```python
from build123d import *
from build123d.topology import SkipClean

# Parameters (mm, degrees)
SKETCH_1_W          = 100
SKETCH_1_H          = 18
SKETCH_1_R          = 2.6
SKETCH_1_R_2        = 2
SKETCH_1_R_3        = 1.5
EXTRUDE_1_DEPTH     = 10
SKETCH_2_W          = 70
SKETCH_2_H          = 18
CUT_EXTRUDE_1_DEPTH = 2
FILLET_1_R          = 1.5
EXTRUDE_3_DEPTH     = 2
SKETCH_4_R          = 4
EXTRUDE_4_DEPTH     = 1
SKETCH_5_R          = 3.38932831
EXTRUDE_5_DEPTH     = 3.2
SKETCH_6_R          = 3.75
EXTRUDE_6_DEPTH     = 3.2
SKETCH_7_R          = 3.75
EXTRUDE_7_DEPTH     = 3.2
SKETCH_8_R          = 3.75
EXTRUDE_8_DEPTH     = 3.2
CUT_EXTRUDE_2_DEPTH = 1
CUT_EXTRUDE_3_DEPTH = 1
CUT_EXTRUDE_4_DEPTH = 1


with BuildPart() as part:
    # Эскиз1 → Вытянуть1 (new body)
    with BuildSketch(Plane.XY):
        with Locations((50, 9)):
            Rectangle(SKETCH_1_W, SKETCH_1_H)
        with Locations((7.5, 9)):
            Circle(SKETCH_1_R, mode=Mode.SUBTRACT)
        with Locations((92.5, 9)):
            Circle(SKETCH_1_R, mode=Mode.SUBTRACT)
        with Locations((20, 4)):
            Circle(SKETCH_1_R_2, mode=Mode.SUBTRACT)
        with Locations((80, 4)):
            Circle(SKETCH_1_R_2, mode=Mode.SUBTRACT)
        with Locations((30, 14)):
            Circle(SKETCH_1_R_3, mode=Mode.SUBTRACT)
        with Locations((70, 14)):
            Circle(SKETCH_1_R_3, mode=Mode.SUBTRACT)
    extrude(amount=EXTRUDE_1_DEPTH)

    # Эскиз2 → Вырез-Вытянуть1 (cut)
    with BuildSketch(Plane(origin=(0, 0, 0), x_dir=(-1, 0, 0), z_dir=(0, 0, -1))):
        with Locations((-50, 9)):
            Rectangle(SKETCH_2_W, SKETCH_2_H)
    extrude(amount=-CUT_EXTRUDE_1_DEPTH, mode=Mode.SUBTRACT)

    # Скругление1
    fillet_1_edges = [part.edges().sort_by_distance(p)[0] for p in [
        (100, 0, 5),
        (0, 0, 5),
        (100, 18, 5),
        (0, 18, 5),
    ]]
    fillet(fillet_1_edges, radius=FILLET_1_R)

    # Эскиз3 → Вытянуть3 (add)
    with BuildSketch(Plane.XY.offset(10)):
        with BuildLine():
            Line((72.692526424, 16.844371856), (82.811526632, 6.845227231))
            ThreePointArc((82.811526632, 6.845227231), (82.845227231, 1.188473368), (77.188473368, 1.154772769))
            Line((77.188473368, 1.154772769), (77.139063674, 1.203597224))
            Line((77.139063674, 1.203597224), (22.860092921, 1.203597224))
            ThreePointArc((22.860092921, 1.203597224), (17.203597224, 1.139907079), (17.139907079, 6.796402776))
            Line((17.139907079, 6.796402776), (26.916385172, 16.795547401))
            ThreePointArc((26.916385172, 16.795547401), (32.572880868, 16.859237546), (32.636571013, 11.20274185))
            Line((32.636571013, 11.20274185), (29.016893244, 7.500623237))
            Line((29.016893244, 7.500623237), (70.766557833, 7.500623237))
            Line((70.766557833, 7.500623237), (67.06947316, 11.153917394))
            ThreePointArc((67.06947316, 11.153917394), (67.035772561, 16.810671257), (72.692526424, 16.844371856))
        make_face()
    extrude(amount=EXTRUDE_3_DEPTH)

    # Эскиз4 → Вытянуть4 (add)
    with SkipClean():  # the faces are left unmerged after this step: merging them gives an invalid solid
        with BuildSketch(Plane.XY.offset(12)):
            with Locations(Location((20, 4, 0), (0, 0, 135.645102996))):
                Circle(SKETCH_4_R)
            with Locations(Location((29.776478092, 13.999144625, 0), (0, 0, 135.645102996))):
                Circle(SKETCH_4_R)
            with Locations(Location((69.880999792, 13.999144625, 0), (0, 0, 225.341340509))):
                Circle(SKETCH_4_R)
            with Locations(Location((80, 4, 0), (0, 0, 225.341340509))):
                Circle(SKETCH_4_R)
        extrude(amount=EXTRUDE_4_DEPTH)
    add(part.part.scale(1), mode=Mode.REPLACE)  # the faces are merged on a copy

    # Эскиз5 → Вытянуть5 (add)
    with BuildSketch(Plane.XY.offset(13)):
        with Locations(Location((80, 4, 0), (0, 0, 143.222791585))):
            Circle(SKETCH_5_R)
    extrude(amount=EXTRUDE_5_DEPTH)

    # Эскиз6 → Вытянуть6 (add)
    with BuildSketch(Plane.XY.offset(13)):
        with Locations(Location((69.880999792, 13.999144625, 0), (0, 0, 141.123198866))):
            Circle(SKETCH_6_R)
    extrude(amount=EXTRUDE_6_DEPTH)

    # Эскиз7 → Вытянуть7 (add)
    with BuildSketch(Plane.XY.offset(13)):
        with Locations(Location((29.776478092, 13.999144625, 0), (0, 0, 141.123198866))):
            Circle(SKETCH_7_R)
    extrude(amount=EXTRUDE_7_DEPTH)

    # Эскиз8 → Вытянуть8 (add)
    with BuildSketch(Plane.XY.offset(13)):
        with Locations(Location((20, 4, 0), (0, 0, 141.123198866))):
            Circle(SKETCH_8_R)
    extrude(amount=EXTRUDE_8_DEPTH)

    # Эскиз9 → Вырез-Вытянуть2 (cut)
    with BuildSketch(Plane.XY.offset(16.2)):
        Polygon((16.157845588, 7.276468987), (24.091280084, -0.656965509), (24.596689062, -0.031003637), (16.723531013, 7.842154412), align=None)
    extrude(amount=-CUT_EXTRUDE_2_DEPTH, mode=Mode.SUBTRACT)

    # Эскиз10 → Вырез-Вытянуть3 (cut)
    with BuildSketch(Plane.XY.offset(16.2)):
        Polygon((23.332366462, 19.877570831), (34.653872269, 8.556065024), (35.333565103, 9.007743039), (23.898051887, 20.443256256), align=None)
    extrude(amount=-CUT_EXTRUDE_3_DEPTH, mode=Mode.SUBTRACT)

    # Эскиз11 → Вырез-Вытянуть4 (cut)
    with BuildSketch(Plane.XY.offset(16.2)):
        Polygon((62.841835451, 20.472623541), (84.739405762, -1.42494677), (85.695784292, -1.249954449), (63.522860335, 20.922969507), align=None)
    extrude(amount=-CUT_EXTRUDE_4_DEPTH, mode=Mode.SUBTRACT)


solid = part.part
```
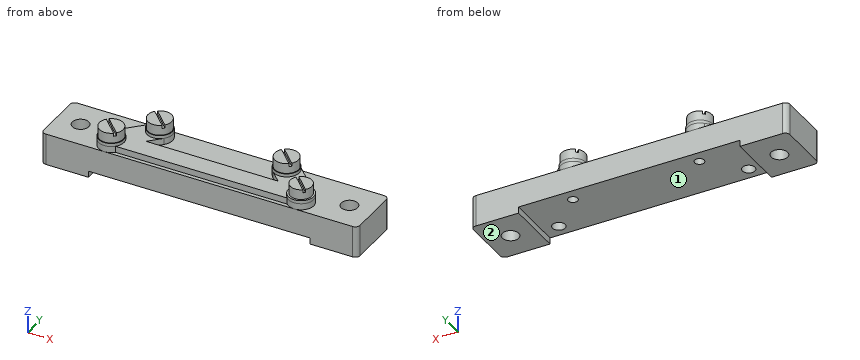
Work out the finished part from the listing and answer in its coordinate system (mm). Face numbers are marked on the shaded views. A direction names the side the tool comes from. Give positions to 0.01 mm unless a question says otherwise; leave off trailing zeros. Write each loop counter-clockwise with the first axis right and the second up, starting at its lowest first coordinate (ties: lowest second). Pieces come first, ordered by that corner, then holes.
(1) Straight lines are drawn through the part: line 1 (X direction, y = 4, z = 8.75); line 2 (X direction, y = 14.25, z = 7.75); line 3 (Y direction, x = 30, z = 6.5). For each, find the intervals that lie inside material, in ascending order.
Final values:
line 1: x = 0 to 18, 22 to 78, 82 to 100
line 2: x = 0 to 28.52, 31.48 to 68.52, 71.48 to 100
line 3: y = 0 to 12.5, 15.5 to 18
(2) Flat-ended cylindrical pins translate along their axes: pin 1 Ø0.9 at (x, y) = (70, 14.5) entering from -Z; pin 2 Ø4.5 at (x, y) = (51.5, 7.5) entering from +Z; pin 3 Ø4.5 at (x, y) = (20.5, 5) entering from -Z. Find the tip coordinate at first contact, or state that the pin passes through.
Final values:
pin 1: stops at z = 10
pin 2: stops at z = 12
pin 3: stops at z = 2
(3) The part is cut by section B-B on z = 8.5. Write down the section's boundary in (x, y), plus the area to 3 significant figures.
Final values:
outline: (0, 1.5) arc R1.5 ccw to (1.5, 0) - (98.5, 0) arc R1.5 ccw to (100, 1.5) - (100, 16.5) arc R1.5 ccw to (98.5, 18) - (1.5, 18) arc R1.5 ccw to (0, 16.5) - close; hole circle Ø5.2 at (7.5, 9); hole circle Ø4 at (20, 4); hole circle Ø3 at (30, 14); hole circle Ø3 at (70, 14); hole circle Ø4 at (80, 4); hole circle Ø5.2 at (92.5, 9)
area: 1,720 mm2
(4) Which of the six approach directions +Z, -Z, +X, -X, +Y, -Y give full straight-line access (tool end or side, diameter ignored) to the marked faces 1 and 2?
Final values:
face 1: -Z, +Y, -Y
face 2: -Z, +X, -X, +Y, -Y
(5) The part is cut by section C-C on x = 41. Write down the section's boundary in (y, z).
Final values:
outline: (0, 2) - (18, 2) - (18, 10) - (7.5, 10) - (7.5, 12) - (1.2, 12) - (1.2, 10) - (0, 10) - close
(6) The part is cut by section A-A on x = 92.5. Write down the section's boundary in (y, z).
Final values:
outline: (0, 0) - (6.4, 0) - (6.4, 10) - (0, 10) - close; (11.6, 0) - (18, 0) - (18, 10) - (11.6, 10) - close
